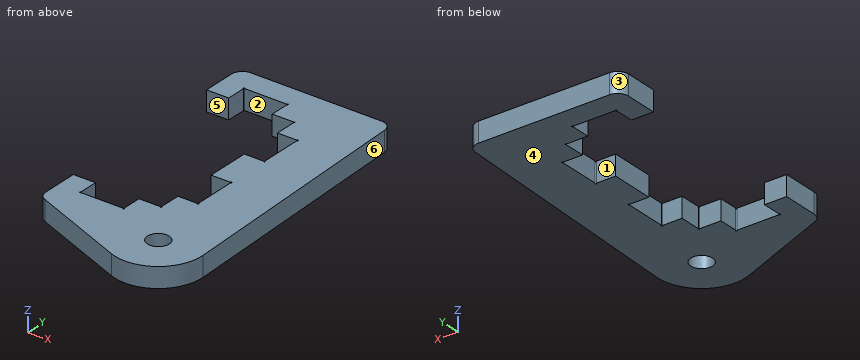
```python
from build123d import *

# Parameters (mm, degrees)
SKETCH1_R           = 3.175
BOSS_EXTRUDE1_DEPTH = 5.842
FILLET2_R           = 3.175
SKETCH2_R           = 0.1984375
CUT_EXTRUDE1_DEPTH  = 63.076766734


with BuildPart() as part:
    # Sketch1 → Boss-Extrude1 (new body)
    with BuildSketch(Plane.XY):
        with BuildLine():
            Line((-12.8, -25.5), (-6.35, -25.5))
            Line((-6.35, -25.5), (-6.35, -31.342))
            Line((-6.35, -31.342), (6.35, -31.342))
            Line((6.35, -31.342), (6.35, -25.5))
            Line((6.35, -25.5), (12.8, -25.5))
            Line((12.8, -25.5), (12.8, -19.05))
            Line((12.8, -19.05), (18.642, -19.05))
            Line((18.642, -19.05), (18.642, -6.35))
            Line((18.642, -6.35), (12.8, -6.35))
            Line((12.8, -6.35), (12.8, 6.35))
            Line((12.8, 6.35), (18.642, 6.35))
            Line((18.642, 6.35), (18.642, 19.05))
            Line((18.642, 19.05), (12.8, 19.05))
            Line((12.8, 19.05), (12.8, 25.5))
            Line((12.8, 25.5), (6.35, 25.5))
            Line((6.35, 25.5), (6.35, 31.342))
            Line((6.35, 31.342), (-6.35, 31.342))
            Line((-6.35, 31.342), (-6.35, 25.5))
            Line((-6.35, 25.5), (-12.8, 25.5))
            Line((-12.8, 25.5), (-12.8, 38.2))
            Line((-12.8, 38.2), (31.65, 38.2))
            Line((31.65, 38.2), (34.596048217, -38.0134839))
            ThreePointArc((34.596048217, -38.0134839), (29.212391738, -48.89151732), (17.154957424, -50.282073297))
            Line((17.154957424, -50.282073297), (-12.8, -38.2))
            Line((-12.8, -38.2), (-12.8, -25.5))
        make_face()
        with Locations((21.905525927, -38.504038703)):
            Circle(SKETCH1_R, mode=Mode.SUBTRACT)
    extrude(amount=BOSS_EXTRUDE1_DEPTH)

    # Fillet2
    fillet2_edges = [part.edges().sort_by_distance(p)[0] for p in [
        (-12.8, 38.2, 2.921),
        (31.65, 38.2, 2.921),
        (-12.8, -38.2, 2.921),
    ]]
    fillet(fillet2_edges, radius=FILLET2_R)

    # Sketch2 → Cut-Extrude1 (cut, through all)
    with BuildSketch(Plane.XY.offset(5.842)):
        with Locations((-6.35, 31.342)):
            Circle(SKETCH2_R)
        with Locations((6.35, 31.342)):
            Circle(SKETCH2_R)
        with Locations((12.8, 25.5)):
            Circle(SKETCH2_R)
        with Locations((18.642, 6.35)):
            Circle(SKETCH2_R)
        with Locations((18.642, 19.05)):
            Circle(SKETCH2_R)
        with Locations((18.642, -19.05)):
            Circle(SKETCH2_R)
        with Locations((18.642, -6.35)):
            Circle(SKETCH2_R)
        with Locations((12.8, -25.5)):
            Circle(SKETCH2_R)
        with Locations((6.35, -31.342)):
            Circle(SKETCH2_R)
        with Locations((-6.35, -31.342)):
            Circle(SKETCH2_R)
    extrude(amount=-CUT_EXTRUDE1_DEPTH, mode=Mode.SUBTRACT)


solid = part.part
```
The model under review builds one solid part; all positions refer to its coordinate system, in mm. Face numbers are marked on the shaded views. A direction names the side the tool comes from. Give positions to 0.01 mm unless a question says otherwise; leave off trailing zeros. Write each loop counter-clockwise with the first axis right and the second up, starting at its lowest first coordinate (ties: lowest second). Pieces come first, ordered by that corner, then holes.
(1) Consider section A-A, the plane y = -40. Give the boundary of the cut face in (x, z), and give its area (3 significant figures).
(2) Consider section C-C, the plane y = 0. Give the boundary of the cut face in (x, z), and give its area (3 significant figures).
(3) Tool access review of the marked faces 1, 2 and 3: name each direction out of +Z, -Z, +X, -X, +Y, -Y from which nothing blocks a thin tool from reaching the whole face with its end or side.
(4) To check wall thickness, follow L1, parallel to Y at x = 4.5, z = 2.25; L2, parallel to Y at x = 10, z = 4.4; L3, parallel to X at y = -39, z = 4.8. State the ranges of each line that lie inside material, in increasing order.
(5) For P1, Ø1.7, axis at x = 16.5, z = 2, coming from the -Y side; P2, Ø1.5, axis at x = 27.5, z = 1.5, coming from the -Y side; P3, Ø3, axis at x = 1, z = 2, coming from the -Y side, all flat-tipped, find the tip position at first contact; note any pin that passes through.
(6) Consider section B-B, the plane y = -13. Give the boundary of the cut face in (x, z).
(7) The part is to be moulded in two halves that separate along Y. For the marked faces 4, 5 and 6, say which applies: released by +Y, released by -Y, zero draft, split by the parting line, or undercut.
Returned:
1. outline: (-8.34, 0) - (19.11, 0) - (19.11, 5.84) - (-8.34, 5.84) - close; (24.71, 0) - (34.52, 0) - (34.52, 5.84) - (24.71, 5.84) - close
1. area: 218 mm2
2. outline: (12.8, 0) - (33.13, 0) - (33.13, 5.84) - (12.8, 5.84) - close
2. area: 119 mm2
3. face 1: +Z, -Z, -X
3. face 2: +Z, -Z
3. face 3: +Z, -Z, -X, +Y
4. L1: y = -45.18 to -31.34, 31.34 to 38.2
4. L2: y = -47.4 to -25.5, 25.5 to 38.2
4. L3: x = -10.82 to 18.77, 25.04 to 34.6
5. P1: stops at y = -50.36
5. P2: stops at y = -50.24
5. P3: stops at y = -44.37
6. outline: (18.64, 0) - (33.63, 0) - (33.63, 5.84) - (18.64, 5.84) - close
7. face 4: zero draft
7. face 5: undercut
7. face 6: released by +Y
